For this review, take the finished solid that the model builds, in its own axes (mm). Give positions to 0.01 mm unless a question says otherwise; leave off trailing zeros. Loops run counter-clockwise (first coordinate to the right, second up) from the corner with the lowest first, then second, coordinate; pieces in that order, holes last.
```python
from build123d import *

# Parameters (mm, degrees)
SKETCH1_W                   = 101.6
SKETCH1_H                   = 101.6
SKETCH1_R                   = 12.7
BOSS_EXTRUDE1_DEPTH         = 6.35
F_1_4_0_25_DIAMETER_HOLE1_D = 6.35
CIRPATTERN1_COUNT           = 4


with BuildPart() as part:
    # Sketch1 → Boss-Extrude1 (new body)
    with BuildSketch(Plane(origin=(0, 0, 0), x_dir=(1, 0, 0), z_dir=(0, 1, 0))):
        Rectangle(SKETCH1_W, SKETCH1_H)
        with Locations(Location((0, 0, 0), (0, 0, 270))):
            Circle(SKETCH1_R, mode=Mode.SUBTRACT)
    extrude(amount=BOSS_EXTRUDE1_DEPTH)

    # 1/4 (0.25) Diameter Hole1 (through all)
    with Locations(Plane(origin=(0, 6.35, 0), x_dir=(1, 0, 0), z_dir=(0, 1, 0))):
        with Locations((-31.75, -31.75)):
            f_1_4_0_25_diameter_hole1 = Hole(F_1_4_0_25_DIAMETER_HOLE1_D / 2)

    # CirPattern1: 1/4 (0.25) Diameter Hole1 ×4 about axis
    cirpattern1_axis = Axis((0, 0, 0), (0, 1, 0))
    for i in range(1, CIRPATTERN1_COUNT):
        add(f_1_4_0_25_diameter_hole1.rotate(cirpattern1_axis, i * 360 / CIRPATTERN1_COUNT), mode=Mode.SUBTRACT)


solid = part.part
```
Item 1: Take a section at A-A on x = 0. Give the boundary of the cut face in (y, z), and give its area (3 significant figures).
Answer:
outline: (0, -50.8) - (6.35, -50.8) - (6.35, -12.7) - (0, -12.7) - close; (0, 12.7) - (6.35, 12.7) - (6.35, 50.8) - (0, 50.8) - close
area: 484 mm2
Item 2: The part is to be moulded in two halves that separate along X. For faces 1 (the flat face through (-12, 6.35, -12)), 2 (the flat face through (-50.8, 3, 1)), 3 (the cylindrical face through (-31.06, 3.13, 34.85)), say which applies: released by +X, released by -X, zero draft, split by the parting line, or undercut.
Answer:
face 1: zero draft
face 2: released by -X
face 3: undercut
Item 3: Take a section at D-D on x = -31.75. Give the boundary of the cut face in (y, z) (3 decimals).
Answer:
outline: (0, -50.8) - (6.35, -50.8) - (6.35, -34.925) - (0, -34.925) - close; (0, -28.575) - (6.35, -28.575) - (6.35, 28.575) - (0, 28.575) - close; (0, 34.925) - (6.35, 34.925) - (6.35, 50.8) - (0, 50.8) - close
Item 4: Take a section at B-B on z = -31.75. Give the boundary of the cut face in (x, y) (3 decimals).
Answer:
outline: (-50.8, 0) - (-34.925, 0) - (-34.925, 6.35) - (-50.8, 6.35) - close; (-28.575, 0) - (28.575, 0) - (28.575, 6.35) - (-28.575, 6.35) - close; (34.925, 0) - (50.8, 0) - (50.8, 6.35) - (34.925, 6.35) - close
Item 5: Clearance check with a flat-ended pin moving along its axis: pin 1 Ø4 at (x, z) = (31.75, -31.75) entering from +Y. State where the tip first meets the part, or that it passes through.
Answer:
pin 1: passes through
Item 6: Take a section at C-C on y = 3. Give the boundary of the cut face in (x, z) (3 decimals), and give its area (3 significant figures).
Answer:
outline: (-50.8, -50.8) - (50.8, -50.8) - (50.8, 50.8) - (-50.8, 50.8) - close; hole circle Ø6.35 at (-31.75, -31.75); hole circle Ø6.35 at (-31.75, 31.75); hole circle Ø25.4 at (0, 0); hole circle Ø6.35 at (31.75, -31.75); hole circle Ø6.35 at (31.75, 31.75)
area: 9,690 mm2
Item 7: For L1, parallel to Z at x = 31.75, y = 3.75 (3 decimals); L2, parallel to Z at x = 31, y = 3, list the stretches that pass through material, from the lowest coordinate up.
Answer:
L1: z = -50.8 to -34.925, -28.575 to 28.575, 34.925 to 50.8
L2: z = -50.8 to -34.84, -28.66 to 28.66, 34.84 to 50.8
